Job drawing, mm, ordinate dimensions from the low corner. One solid piece. A direction names the side the tool comes from. Give positions to 0.01 mm unless a question says otherwise; leave off trailing zeros. Loops run counter-clockwise (first coordinate to the right, second up) from the corner with the lowest first, then second, coordinate; pieces in that order, holes last. Notation, with made-up numbers: M 8.5,48 L 57.5,48 A18 cw 57.5,71 Z; hole C 11.25,-20.75 d6. An arc over 180 degrees is marked long. Answer as CSV lines item,"result".
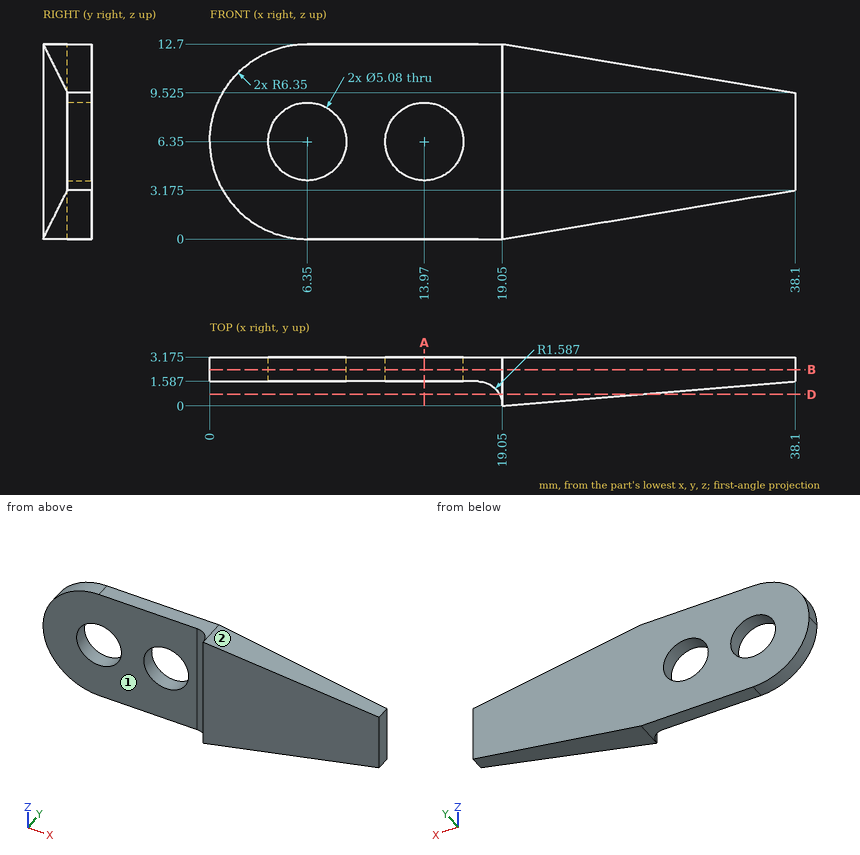
1) Band-saw the part on B-B on y = 2.35. Give the number of separate pieces and of enclosed holes in the cut face.
Answer below:
separate pieces,"1"
enclosed holes,"2"
2) Band-saw the part on D-D on y = 0.75. Give the cut face in (x, z).
Answer below:
outline,"M 18.86,0 L 19.05,0 L 28.05,1.5 L 28.05,11.2 L 19.05,12.7 L 18.86,12.7 Z"
3) Band-saw the part on A-A on x = 13.97. Give the cut face in (y, z) (1 decimal).
Answer below:
outline,"M 1.6,0 L 3.2,0 L 3.2,3.8 L 1.6,3.8 Z; M 1.6,8.9 L 3.2,8.9 L 3.2,12.7 L 1.6,12.7 Z"
4) Flat gauge pins, fed straight in: pin 1 (1.5 mm diameter, centred on y = 1, z = 10.5, fed in from -X); pin 2 (6.5 mm diameter, centred on x = 10, z = 4.5, fed in from -Y). Where does each tip first touch, or does it go through?
Answer below:
pin 1,"stops at x = 1.18"
pin 2,"stops at y = 1.59"
5) Which spindle directions (+Z, -Z, +X, -X, +Y, -Y) get a long thin tool onto all of the face, cutting with end or side? Do the marked faces 1 and 2. Say none if no direction does.
Answer below:
face 1,"+Z, -Z, -X, -Y"
face 2,"+Z, +X, +Y, -Y"
6) Drill centre lines: line 1 (X direction, y = 2.4, z = 6.35); line 2 (X direction, y = 2.7, z = 7.5) (1 decimal); line 3 (Y direction, x = 7, z = 10.5) (1 decimal). Where is each one in solid material? Low to high. Write a range as from..to.
Answer below:
line 1,"x = 0..3.81, 8.89..11.43, 16.51..38.1"
line 2,"x = 0.1..4.1, 8.6..11.7, 16.2..38.1"
line 3,"y = 1.6..3.2"
